```python
from build123d import *

# Parameters (mm, degrees)
SKETCH1_W           = 16
SKETCH1_H           = 6
SKETCH1_R           = 1.5
BOSS_EXTRUDE1_DEPTH = 0.5
BOSS_EXTRUDE2_DEPTH = 16
SKETCH3_R           = 1.5
CUT_EXTRUDE1_DEPTH  = 8.659646886
SKETCH4_W           = 16
SKETCH4_H           = 8
BOSS_EXTRUDE3_DEPTH = 0.5


with BuildPart() as part:
    # Sketch1 → Boss-Extrude1 (new body)
    with BuildSketch(Plane.XY):
        Rectangle(SKETCH1_W, SKETCH1_H)
        with Locations((-4.5, 0)):
            Circle(SKETCH1_R, mode=Mode.SUBTRACT)
        with Locations((4.5, 0)):
            Circle(SKETCH1_R, mode=Mode.SUBTRACT)
    extrude(amount=BOSS_EXTRUDE1_DEPTH)

    # Sketch2 → Boss-Extrude2 (add)
    with BuildSketch(Plane.ZY.offset(8)):
        with BuildLine():
            ThreePointArc((0.163996883, 18.220231427), (0.415988989, 10.611969896), (0.5, 3))
            Line((0.5, 3), (0, 3))
            ThreePointArc((0, 3), (-0.083889217, 10.600934542), (-0.335516001, 18.198166096))
            ThreePointArc((-0.335516001, 18.198166096), (-0.36155667, 24.039453598), (0.075644223, 29.864414815))
            Line((0.075644223, 29.864414815), (1.666879953, 43.688343289))
            Line((1.666879953, 43.688343289), (1.914976685, 45.843694255))
            Line((1.914976685, 45.843694255), (3.506212415, 59.667622728))
            Line((3.506212415, 59.667622728), (4.002932547, 59.610446591))
            Line((4.002932547, 59.610446591), (0.572364355, 29.807238679))
            ThreePointArc((0.572364355, 29.807238679), (0.138133092, 24.021842748), (0.163996883, 18.220231427))
        make_face()
    extrude(amount=-BOSS_EXTRUDE2_DEPTH)

    # Sketch3 → Cut-Extrude1 (cut, through all)
    with BuildSketch(Plane(origin=(0, 0.381926952, -3.318006735), x_dir=(-1, 0, 0), z_dir=(0, 0.114352273, -0.993440264))):
        with Locations((-4.5, 44.67716222)):
            Circle(SKETCH3_R)
        with Locations((4.5, 44.67716222)):
            Circle(SKETCH3_R)
    extrude(amount=-CUT_EXTRUDE1_DEPTH, mode=Mode.SUBTRACT)

    # Sketch4 → Boss-Extrude3 (add)
    with BuildSketch(Plane(origin=(0, 0.381926952, -3.318006735), x_dir=(-1, 0, 0), z_dir=(0, 0.114352273, -0.993440264))):
        with Locations((0, 63.67716222)):
            Rectangle(SKETCH4_W, SKETCH4_H)
    extrude(amount=-BOSS_EXTRUDE3_DEPTH)


solid = part.part
```
CAD build for the part. Positions are in the model's coordinates, mm. A direction names the side the tool comes from. Coordinates: 2 decimals unless noted, no trailing zeros. Write each loop counter-clockwise with the first axis right and the second up, starting at its lowest first coordinate (ties: lowest second). Pieces come first, ordered by that corner, then holes. Notation, with made-up numbers: (51.25, 28.25) -> (61.25, 28.25) arc R25 cw to (61.25, 42.25) -> close; hole circle Ø10 at (32, 21.25). An arc over 180 degrees is marked (long way). Return JSON: item names as keys, results as strings. Group by question number.
Q1. Cut at A-A, the plane y = 0. Give the cut face in (x, z).
Q2. Drill centre lines: line 1 (Z direction, x = -3.25, y = 1.5); line 2 (Z direction, x = 6, y = 18). Where is each one in solid material? Low to high.
Q3. Which spindle directions (+Z, -Z, +X, -X, +Y, -Y) get a long thin tool onto all of the face, cutting with end or side? Do faces 4 (the face through (0, 0, 0)), 5 (the face through (0, 0, 0.5)), 6 (the face through (-0.112, 10.719, 0.414)), 7 (the face through (-5.31, 45.99, 2.18)). Say none if no direction does.
Q4. Cut at C-C, the plane x = -6.75. Give the cut face in (y, z), then the cut area to 3 significant figures.
Q5. Cut at D-D, the plane y = 40. Give the cut face in (x, z).
Q6. Cut at B-B, the plane x = 4.5. Give the cut face in (y, z), then the cut area to 3 significant figures.
Q7. Flat gauge pins, fed straight in: pin 1 (3 mm diameter, centred on x = 1.5, y = -0.5, fed in from +Z); pin 2 (4 mm diameter, centred on x = 5.5, y = 48.5, fed in from +Z); pin 3 (6 mm diameter, centred on x = -5, y = 35, fed in from +Z); pin 4 (1.5 mm diameter, centred on y = 31, z = 0, fed in from -X). Where does each tip first touch, or does it go through?
Q8. Pull direction X, two halves, no side cores. Call faces 1 (the face through (-0.112, 23.958, -0.364)), 2 (the face through (4.695, 46.215, 2.206)), 3 (the face through (-8, 32.3, 0.7)): released by +X, released by -X, zero draft, split by the parting line, or undercut.
Returned:
{
 "1": {"outline": "(-8, 0) -> (-6, 0) -> (-6, 0.5) -> (-8, 0.5) -> close; (-3, 0) -> (3, 0) -> (3, 0.5) -> (-3, 0.5) -> close; (6, 0) -> (8, 0) -> (8, 0.5) -> (6, 0.5) -> close"},
 "2": {"line 1": "z = 0 to 0.5", "line 2": "z = -0.33 to 0.17"},
 "3": {"face 4": "-Z, +X, -X, -Y", "face 5": "+Z, +X, -X, -Y", "face 6": "+Z, +X, -X", "face 7": "none"},
 "4": {"outline": "(-3, 0) -> (3, 0) arc R344.39 cw to (18.2, -0.34) arc R73.61 ccw to (29.86, 0.08) -> (67.62, 4.42) -> (67.56, 4.92) -> (29.81, 0.57) arc R73.11 cw to (18.22, 0.16) arc R344.89 ccw to (3, 0.5) -> (-3, 0.5) -> close", "area": "35.4 mm2"},
 "5": {"outline": "(-8, 1.24) -> (8, 1.24) -> (8, 1.75) -> (-8, 1.75) -> close"},
 "6": {"outline": "(-3, 0) -> (-1.5, 0) -> (-1.5, 0.5) -> (-3, 0.5) -> close; (1.5, 0) -> (3, 0) arc R344.39 cw to (18.2, -0.34) arc R73.61 ccw to (29.86, 0.08) -> (43.28, 1.62) -> (43.22, 2.12) -> (29.81, 0.57) arc R73.11 cw to (18.22, 0.16) arc R344.89 ccw to (3, 0.5) -> (1.5, 0.5) -> close; (46.2, 2.46) -> (46.26, 1.96) -> (67.62, 4.42) -> (67.56, 4.92) -> close", "area": "32.4 mm2"},
 "7": {"pin 1": "stops at z = 0.5", "pin 2": "stops at z = 2.95", "pin 3": "stops at z = 1.52", "pin 4": "stops at x = -8"},
 "8": {"face 1": "zero draft", "face 2": "undercut", "face 3": "released by -X"}
}
